```python
from build123d import *

# Parameters (mm, degrees)
SKETCH_1_R      = 1.6
SKETCH_1_R_2    = 0.5
SKETCH_1_W      = 9
SKETCH_1_H      = 5
EXTRUDE_1_DEPTH = 2


with BuildPart() as part:
    # 草图1 → 凸台-拉伸1 (new body)
    with BuildSketch(Plane(origin=(0, 0, 0), x_dir=(1, 0, 0), z_dir=(0, 1, 0))):
        with BuildLine():
            Line((-15.25, -18), (15.25, -18))
            ThreePointArc((15.25, -18), (17.194543648, -17.194543648), (18, -15.25))
            Line((18, -15.25), (18, 15.25))
            ThreePointArc((18, 15.25), (17.194543648, 17.194543648), (15.25, 18))
            Line((15.25, 18), (-15.25, 18))
            ThreePointArc((-15.25, 18), (-17.194543648, 17.194543648), (-18, 15.25))
            Line((-18, 15.25), (-18, -15.25))
            ThreePointArc((-18, -15.25), (-17.194543648, -17.194543648), (-15.25, -18))
        make_face()
        with Locations(Location((15.25, 15.25, 0), (0, 0, 270))):
            Circle(SKETCH_1_R, mode=Mode.SUBTRACT)
        with Locations(Location((15.25, -15.25, 0), (0, 0, 270))):
            Circle(SKETCH_1_R, mode=Mode.SUBTRACT)
        with Locations(Location((-15.25, -15.25, 0), (0, 0, 270))):
            Circle(SKETCH_1_R, mode=Mode.SUBTRACT)
        with Locations(Location((-15.25, 15.25, 0), (0, 0, 270))):
            Circle(SKETCH_1_R, mode=Mode.SUBTRACT)
        with Locations(Location((-6.5, 0, 0), (0, 0, 270))):
            Circle(SKETCH_1_R_2, mode=Mode.SUBTRACT)
        with Locations(Location((6.5, 0, 0), (0, 0, 90))):
            Circle(SKETCH_1_R_2, mode=Mode.SUBTRACT)
        with Locations((0, -7)):
            Rectangle(SKETCH_1_W, SKETCH_1_H, mode=Mode.SUBTRACT)
    extrude(amount=EXTRUDE_1_DEPTH)


solid = part.part
```
Source: CAD feature listing. Evaluate the final solid. Frame: model axes, mm. A direction names the side the tool comes from. Round coordinates to 2 decimals unless told otherwise and drop trailing zeros. Loops run counter-clockwise (first coordinate to the right, second up) from the corner with the lowest first, then second, coordinate; pieces in that order, holes last.
1. Contact query for a flat-ended pin moving along its axis: pin 1 (3 mm diameter, centred on x = -15.25, z = 15.25, fed in from -Y). Output: stop coordinate, or through.
2. Section query B-B on x = -6.5. Output: boundary loops of the cut face in (y, z).
3. Section query A-A on z = 0. Output: boundary loops of the cut face in (x, y).
4. Ray query, L1, parallel to X at y = 0.8, z = 0; L2, parallel to X at y = 0.25, z = -15; L3, parallel to Z at x = 14, y = 1.45. Return the intervals inside material, ascending.
5. Mould query, pull axis Z, two halves, no side actions, for faces 1 (the cylindrical face through (17.17, 0.99, 17.22)), 2 (the flat face through (0, 1, 4.5)), 3 (the cylindrical face through (-17.17, 0.99, -17.22)), 4 (the cylindrical face through (-7, 1, 0)). Classes: released by +Z, released by -Z, zero draft, split by the parting line, or undercut.
6. Section query C-C on x = 3. Output: boundary loops of the cut face in (y, z).
7. Access query for faces 5 (the flat face through (-18, 1, 0)), 6 (the flat face through (0, 1, 9.5)). Directions: +Z, -Z, +X, -X, +Y, -Y. A direction counts if a zero-diameter tool reaches every point of the face in a straight line with its end or side. Return the directions, or none.
Answers below:
1. pin 1: passes through
2. outline: (0, -18) - (2, -18) - (2, -0.5) - (0, -0.5) - close; (0, 0.5) - (2, 0.5) - (2, 18) - (0, 18) - close
3. outline: (-18, 0) - (-7, 0) - (-7, 2) - (-18, 2) - close; (-6, 0) - (6, 0) - (6, 2) - (-6, 2) - close; (7, 0) - (18, 0) - (18, 2) - (7, 2) - close
4. L1: x = -18 to -7, -6 to 6, 7 to 18
4. L2: x = -18 to -16.83, -13.67 to 13.67, 16.83 to 18
4. L3: z = -18 to -16.25, -14.25 to 14.25, 16.25 to 18
5. face 1: released by +Z
5. face 2: undercut
5. face 3: released by -Z
5. face 4: undercut
6. outline: (0, -18) - (2, -18) - (2, 4.5) - (0, 4.5) - close; (0, 9.5) - (2, 9.5) - (2, 18) - (0, 18) - close
7. face 5: +Z, -Z, -X, +Y, -Y
7. face 6: +Y, -Y
